```python
from build123d import *

# Parameters (mm, degrees)
SKETCH2_W           = 106
SKETCH2_H           = 2
BOSS_EXTRUDE1_DEPTH = 72
SKETCH4_R           = 1.325
CUT_EXTRUDE1_DEPTH  = 90.425947018
SKETCH6_W           = 38.22100301
SKETCH6_H           = 41.408309334
CUT_EXTRUDE3_DEPTH  = 10
SKETCH5_R           = 1.7
BOSS_EXTRUDE2_DEPTH = 1.92


with BuildPart() as part:
    # Sketch2 → Boss-Extrude1 (new body)
    with BuildSketch(Plane.XY):
        Rectangle(SKETCH2_W, SKETCH2_H)
    extrude(amount=BOSS_EXTRUDE1_DEPTH)

    # Sketch4 → Cut-Extrude1 (cut, through all)
    with BuildSketch(Plane(origin=(0, 1, 0), x_dir=(1, 0, 0), z_dir=(0, 1, 0))):
        with Locations(Location((-50.004878073, -6.450693227, 0), (0, 0, 270))):
            Circle(SKETCH4_R)
        with Locations(Location((-50.004878073, -68.250693227, 0), (0, 0, 270))):
            Circle(SKETCH4_R)
        with Locations(Location((49.295121927, -68.250693227, 0), (0, 0, 270))):
            Circle(SKETCH4_R)
        with Locations(Location((49.295121927, -6.450693227, 0), (0, 0, 270))):
            Circle(SKETCH4_R)
    extrude(amount=-CUT_EXTRUDE1_DEPTH, mode=Mode.SUBTRACT)

    # Sketch6 → Cut-Extrude3 (cut)
    with BuildSketch(Plane(origin=(0, 1, 0), x_dir=(1, 0, 0), z_dir=(0, 1, 0))):
        with Locations((23, -36)):
            Rectangle(SKETCH6_W, SKETCH6_H)
    extrude(amount=-CUT_EXTRUDE3_DEPTH, mode=Mode.SUBTRACT)

    # Sketch5 → Boss-Extrude2 (add)
    with BuildSketch(Plane(origin=(0, 0, 0), x_dir=(-1, 0, 0), z_dir=(0, 0, -1))):
        with Locations(Location((0, 0, 0), (0, 0, 216.031879072))):
            Circle(SKETCH5_R)
        with Locations(Location((26.5, 0, 0), (0, 0, 143.968120928))):
            Circle(SKETCH5_R)
        with Locations(Location((-26.5, 0, 0), (0, 0, 143.968120928))):
            Circle(SKETCH5_R)
    extrude(amount=BOSS_EXTRUDE2_DEPTH)


solid = part.part
```
The model under review builds one solid part; all positions refer to its coordinate system, in mm. A direction names the side the tool comes from. Round coordinates to 2 decimals unless told otherwise and drop trailing zeros. Write each loop counter-clockwise with the first axis right and the second up, starting at its lowest first coordinate (ties: lowest second). Pieces come first, ordered by that corner, then holes. Notation, with made-up numbers: (77.5, 13.5) - (131.5, 13.5) arc R18 cw to (131.5, 37.5) - close; hole circle Ø3 at (-26.75, 78.25). An arc over 180 degrees is marked (long way). Answer as CSV lines item,"result". Start each with the question number.
(1) For faces 4 (the cylindrical face through (28.11, 0.54, -0.95)), 5 (the flat face through (23, 0, 56.704)), 6 (the flat face through (-1, 0, 72)), list the 3-axis set-ups (+Z, -Z, +X, -X, +Y, -Y) from which the entire face can be reached by the end or side of a thin tool; tool diameter is ignored.
(2) To check wall thickness, follow line 1 (Z direction, x = 42, y = 0.6); line 2 (X direction, y = -0.35, z = 50); line 3 (Z direction, x = 48.5, y = -0.6). State the ranges of each line that lie inside material, in increasing order.
(3) Draft analysis for pull direction Z (two halves, no side actions). For faces 1 (the flat face through (-13, 0, 0)), 2 (the flat face through (-1, -1, 35)), 3 (the flat face through (42.111, 0, 36)), state which applies: pulls with the +Z half, pulls with the -Z half, needs draft (parallel to the pull), parting line crosses it, or undercut.
(4) We need section B-B on y = 0.05. Give the number of separate pieces and of enclosed holes in the cut face, plus the area to 3 significant figures.
(5) We need section A-A on x = 26.5. State the section outline as (y, z) points, plus the area to 3 significant figures.
(6) We need section C-C on x = 0. State the section outline as (y, z) points, plus the area to 3 significant figures.
(7) For pin 1 Ø2 at (x, y) = (-39.5, -1.5) entering from -Z; pin 2 Ø8 at (x, z) = (-28.5, 18) entering from -Y; pin 3 Ø0.6 at (x, y) = (-26.5, -1.5) entering from +Z; pin 4 Ø2 at (x, z) = (49.3, 6.45) entering from +Y, all flat-tipped, find the tip position at first contact; note any pin that passes through.
(8) We need section D-D on z = 12.5. State the section outline as (x, y) points.
Worked answers:
1,face 4,"-Z"
1,face 5,"+Y, -Y"
1,face 6,"+Z, +X, -X, +Y, -Y"
2,line 1,"0 to 15.3, 56.7 to 72"
2,line 2,"-53 to 3.89, 42.11 to 53"
2,line 3,"0 to 5.39, 7.51 to 67.19, 69.31 to 72"
3,face 1,"pulls with the -Z half"
3,face 2,"needs draft"
3,face 3,"undercut"
4,separate pieces,"1"
4,enclosed holes,"5"
4,area,"6,050 mm²"
5,outline,"(-1.7, -1.92) - (1.7, -1.92) - (1.7, 0) - (1, 0) - (1, 15.3) - (-1, 15.3) - (-1, 0) - (-1.7, 0) - close; (-1, 56.7) - (1, 56.7) - (1, 72) - (-1, 72) - close"
5,area,"67.7 mm²"
6,outline,"(-1.7, -1.92) - (1.7, -1.92) - (1.7, 0) - (1, 0) - (1, 72) - (-1, 72) - (-1, 0) - (-1.7, 0) - close"
6,area,"151 mm²"
7,pin 1,"z = 0"
7,pin 2,"y = -1"
7,pin 3,"z = 0"
7,pin 4,"through"
8,outline,"(-53, -1) - (53, -1) - (53, 1) - (-53, 1) - close"
